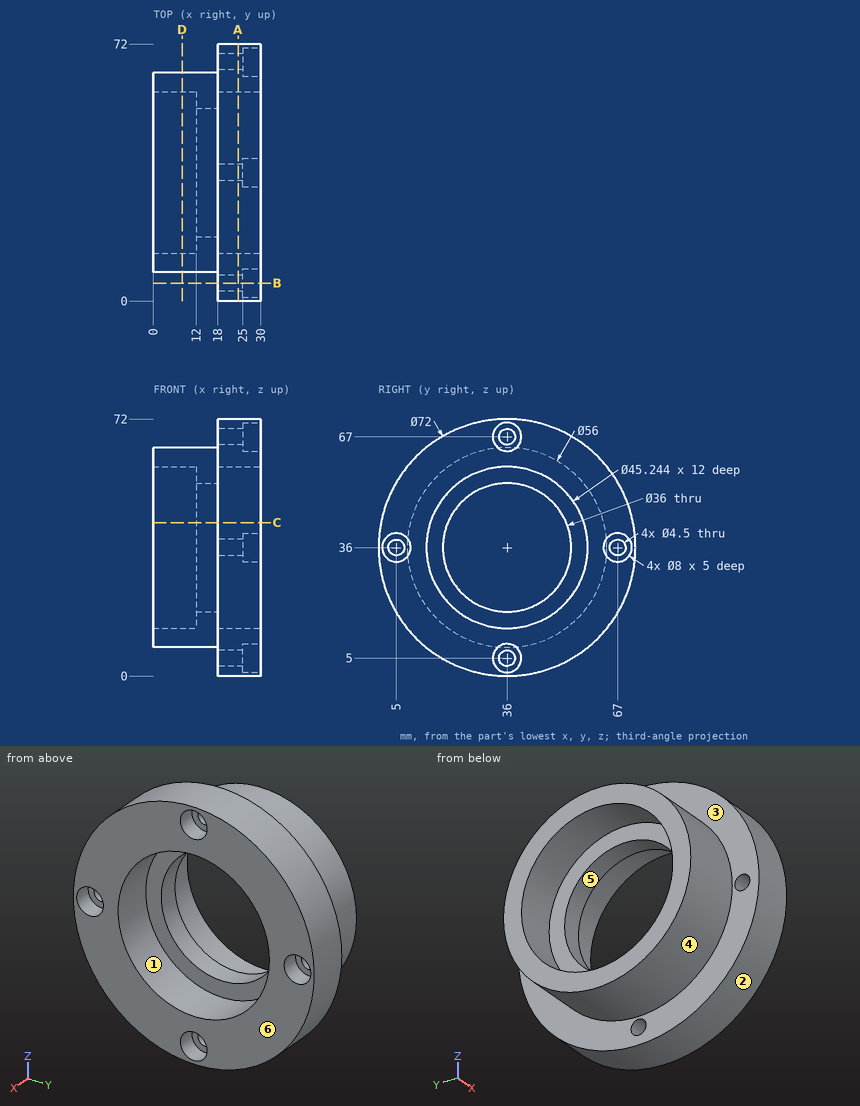
Study the drawing (mm; zero at the part's minimum x, y, z) and answer. A direction names the side the tool comes from. Give positions to 0.01 mm unless a question says otherwise; leave off trailing zeros. Write each loop counter-clockwise with the first axis right and the second up, starting at its lowest first coordinate (ties: lowest second). Pieces come first, ordered by that corner, then holes. Notation, with made-up numbers: (72, 88) -> (112, 88) arc R24 ccw to (112, 117) -> close; hole circle Ø7 at (29.25, 14.25). An arc over 180 degrees is marked (long way). Answer in a Markdown table with one row per item.
1) Section C-C on z = 43 is taken. Give the vertices of the cut face in (x, y), plus the area to 3 significant figures.
Results list:
| item | result |
|---|---|
| outline | (0, 8.89) -> (18, 8.89) -> (18, 0.69) -> (30, 0.69) -> (30, 14.49) -> (18, 14.49) -> (18, 19.42) -> (12, 19.42) -> (12, 14.49) -> (0, 14.49) -> close; (0, 57.51) -> (12, 57.51) -> (12, 52.58) -> (18, 52.58) -> (18, 57.51) -> (30, 57.51) -> (30, 71.31) -> (18, 71.31) -> (18, 63.11) -> (0, 63.11) -> close |
| area | 592 mm^2 |
2) Each of these flat-tipped pins is pushed along its axis until it touches: pin 1 Ø4 at (y, z) = (5, 36) entering from +X (3 decimals); pin 2 Ø5 at (x, y) = (5, 14) entering from +Z; pin 3 Ø2.5 at (y, z) = (5.5, 34.5) entering from +X; pin 4 Ø1 at (y, z) = (14.5, 31) entering from +X. Where does it stop, or does it pass through?
Results list:
| item | result |
|---|---|
| pin 1 | through |
| pin 2 | z = 56.09 |
| pin 3 | x = 25 |
| pin 4 | x = 18 |
3) A tool of negligible diameter and unlimited length cuts with its end or side. For the marked faces 1, 2 and 3, from which of +Z, -Z, +X, -X, +Y, -Y can it reach the whole face along a straight path? Write none if from no direction.
Results list:
| item | result |
|---|---|
| face 1 | +X |
| face 2 | +X, -X |
| face 3 | -X |
4) Straight lines are drawn through the part: line 1 (Z direction, x = 22.75, y = 36); line 2 (Z direction, x = 26.55, y = 36); line 3 (X direction, y = 16.5, z = 35). For each, find the intervals that lie inside material, in ascending order. Write a range as [from, to].
Results list:
| item | result |
|---|---|
| line 1 | [0, 2.75], [7.25, 13.38], [58.62, 64.75], [69.25, 72] |
| line 2 | [0, 1], [9, 13.38], [58.62, 63], [71, 72] |
| line 3 | [12, 18] |
5) Determine the mould class of the marked faces 4, 5 and 6 for opening direction Y: released by +Y, released by -Y, zero draft, split by the parting line, or undercut.
Results list:
| item | result |
|---|---|
| face 4 | split by the parting line |
| face 5 | undercut |
| face 6 | zero draft |
6) Section D-D on x = 8 is taken. Give the vertices of the cut face in (y, z), plus the area to 3 significant figures.
Results list:
| item | result |
|---|---|
| outline | circle Ø56 at (36, 36); hole circle Ø45.24 at (36, 36) |
| area | 855 mm^2 |
7) Section B-B on y = 5 is taken. Give the vertices of the cut face in (x, z), plus the area to 3 significant figures.
Results list:
| item | result |
|---|---|
| outline | (18, 17.7) -> (30, 17.7) -> (30, 32) -> (25, 32) -> (25, 33.75) -> (18, 33.75) -> close; (18, 38.25) -> (25, 38.25) -> (25, 40) -> (30, 40) -> (30, 54.3) -> (18, 54.3) -> close |
| area | 368 mm^2 |
8) Section A-A on x = 23.75 is taken. Give the vertices of the cut face in (y, z), plus the area to 3 significant figures.
Results list:
| item | result |
|---|---|
| outline | circle Ø72 at (36, 36); hole circle Ø4.5 at (5, 36); hole circle Ø45.24 at (36, 36); hole circle Ø4.5 at (36, 5); hole circle Ø4.5 at (36, 67); hole circle Ø4.5 at (67, 36) |
| area | 2,400 mm^2 |
